For this review, use the dimensioned drawing (mm, ordinates from the lowest corner) and the shaded views. A direction names the side the tool comes from. Coordinates: 2 decimals unless noted, no trailing zeros. Order: outer loops, then holes, each group sorted by start corner. A loop starts at its lowest first (then second) coordinate and runs counter-clockwise, first axis right, second up. Notation, with made-up numbers: M 20,-22.5 L 66,-22.5 A20 ccw 66,-1.5 Z; hole C 70.25,22.5 d4. An arc over 180 degrees is marked long. Answer in a Markdown table with one row per item.
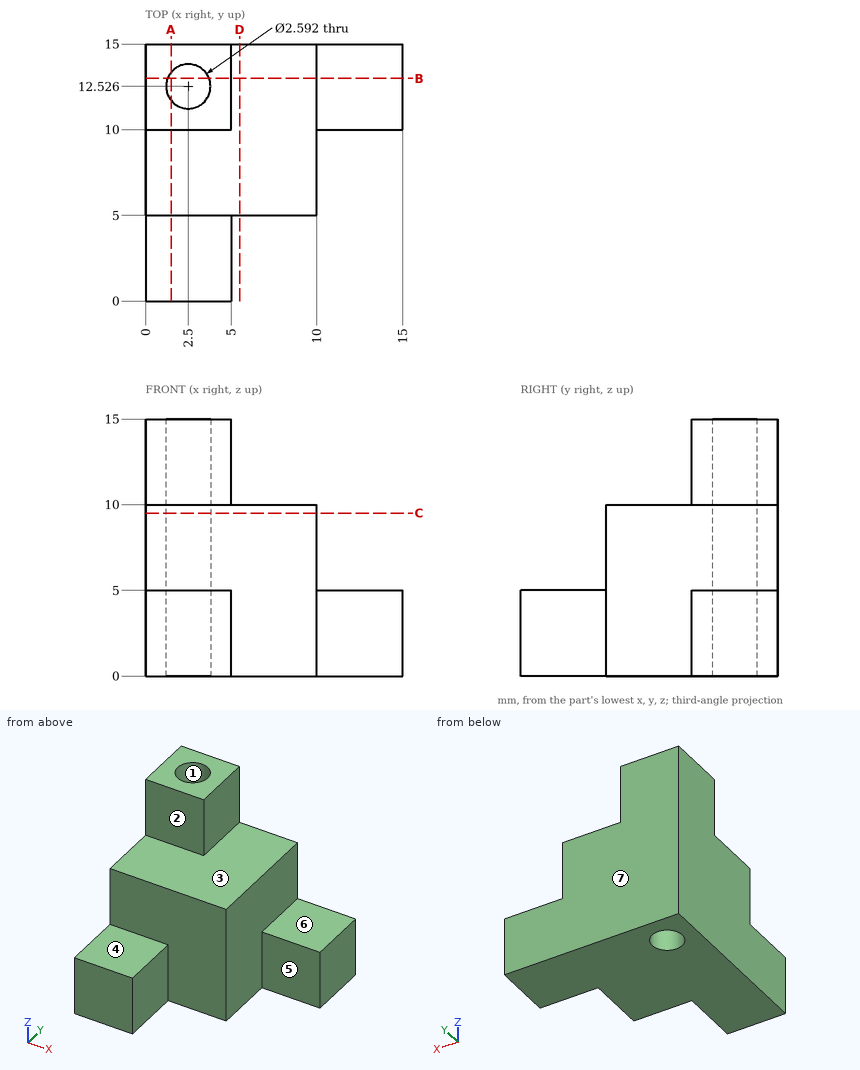
(1) Draft analysis for pull direction Y (two halves, no side actions). For the marked faces 1, 2 and 3, state which applies: pulls with the +Y half, pulls with the -Y half, needs draft (parallel to the pull), parting line crosses it, or undercut.
Return value:
| item | result |
|---|---|
| face 1 | undercut |
| face 2 | pulls with the -Y half |
| face 3 | needs draft |
(2) Add section C-C, the plane z = 9.5. Give the boundary of the cut face in (x, y) (1 decimal).
Return value:
| item | result |
|---|---|
| outline | M 0,5 L 10,5 L 10,15 L 0,15 Z; hole C 2.5,12.5 d2.6 |
(3) Insertion check: pin 1 Ø4 at (y, z) = (1.5, 3) entering from +X; pin 2 Ø5.5 at (x, z) = (3, 12) entering from -Y; pin 3 Ø1.5 at (x, z) = (13, 1.5) entering from -Y. Each pin has a flat end and moves straight along its axis. Give the tip position at first contact, or say it passes through.
Return value:
| item | result |
|---|---|
| pin 1 | stops at x = 5 |
| pin 2 | stops at y = 5 |
| pin 3 | stops at y = 10 |
(4) Add section B-B, the plane y = 13. Give the boundary of the cut face in (x, z).
Return value:
| item | result |
|---|---|
| outline | M 0,0 L 1.29,0 L 1.29,15 L 0,15 Z; M 3.71,0 L 15,0 L 15,5 L 10,5 L 10,10 L 5,10 L 5,15 L 3.71,15 Z |
(5) For the marked faces 4, 5, 6 and 7, list the 3-axis set-ups (+Z, -Z, +X, -X, +Y, -Y) from which the entire face can be reached by the end or side of a thin tool; tool diameter is ignored.
Return value:
| item | result |
|---|---|
| face 4 | +Z, +X, -X, -Y |
| face 5 | +Z, -Z, +X, -Y |
| face 6 | +Z, +X, +Y, -Y |
| face 7 | +Z, -Z, +X, -X, +Y |
(6) Add section A-A, the plane x = 1.5. Give the boundary of the cut face in (y, z), and give its area (3 significant figures).
Return value:
| item | result |
|---|---|
| outline | M 0,0 L 11.7,0 L 11.7,15 L 10,15 L 10,10 L 5,10 L 5,5 L 0,5 Z; M 13.35,0 L 15,0 L 15,15 L 13.35,15 Z |
| area | 125 mm2 |
(7) For line 1 along Y through (x, z) = (2.5, 4.5); line 2 along Y through (x, z) = (2.5, 10.5); line 3 along Z through (x, y) = (12, 11.75), list the stretches that pass through material, from the lowest coordinate up. Write a range as from..to.
Return value:
| item | result |
|---|---|
| line 1 | y = 0..11.23, 13.82..15 |
| line 2 | y = 10..11.23, 13.82..15 |
| line 3 | z = 0..5 |
(8) Add section D-D, the plane x = 5.5. Give the boundary of the cut face in (y, z), and give its area (3 significant figures).
Return value:
| item | result |
|---|---|
| outline | M 5,0 L 15,0 L 15,10 L 5,10 Z |
| area | 100 mm2 |
